Work out the finished part from the listing and answer in its coordinate system (mm). Coordinates: 2 decimals unless noted, no trailing zeros. Write each loop counter-clockwise with the first axis right and the second up, starting at its lowest first coordinate (ties: lowest second). Pieces come first, ordered by that corner, then holes. Notation, with made-up numbers: M 89,-22.5 L 104,-22.5 A20 cw 104,-3.5 Z; hole C 33,85 d10. An arc over 180 degrees is marked long. Answer as CSV lines item,"result". Start each with the question number.
(1) A cutting plane is placed at D-D on x = 0. Give the vertices of the cut face in (y, z), then the cut area to 3 significant figures.
(2) A cutting plane is placed at B-B on y = 22.5. Give the vertices of the cut face in (x, z).
(3) A cutting plane is placed at C-C on z = 1. Count the separate pieces of the cut face and the enclosed holes in it, then the cut area to 3 significant figures.
(4) A cutting plane is placed at A-A on x = 15.5. Give the vertices of the cut face in (y, z).
(5) Find the intervals of material crossed by L1, parallel to X at y = 25, z = 0.15; L2, parallel to Y at x = 15.5, z = 0.9; L3, parallel to Y at x = -25.5, z = 1.95, in increasing order. Write a range as [from, to].
(6) A flat-ended cylindrical pin translates along its axis: P1, Ø2, axis at x = 15.5, y = 15.5, coming from the +Z side. Find the tip coordinate at first contact, or state that the pin passes through.
from build123d import *

# Parameters (mm, degrees)
SKIZZE1_W                        = 70
SKIZZE1_H                        = 70
AUFSATZ_LINEAR_AUSTRAGEN1_DEPTH  = 2
VERRUNDUNG2_R                    = 2
F_23_0_23_DURCHMESSER_BOHRUNG1_D = 23
DURCHGANGSLOCH_F_R_M31_D         = 3.4
SCHNITT_LINEAR_AUSTRAGEN1_DEPTH  = 50.537864306


with BuildPart() as part:
    # Skizze1 → Aufsatz-Linear austragen1 (new body)
    with BuildSketch(Plane.XY):
        Rectangle(SKIZZE1_W, SKIZZE1_H)
    extrude(amount=AUFSATZ_LINEAR_AUSTRAGEN1_DEPTH)

    # Verrundung2
    verrundung2_edges = [part.edges().sort_by_distance(p)[0] for p in [
        (-35, 35, 1),
        (35, 35, 1),
        (35, -35, 1),
        (-35, -35, 1),
    ]]
    fillet(verrundung2_edges, radius=VERRUNDUNG2_R)

    # Ø23.0 (23) Durchmesser Bohrung1 (through all)
    with Locations(Plane.XY.offset(2)):
        with Locations((0, 0)):
            Hole(F_23_0_23_DURCHMESSER_BOHRUNG1_D / 2)

    # Durchgangsloch für M31 (through all)
    with Locations(Plane.XY.offset(2)):
        with Locations((-15.5, 15.5), (15.5, 15.5), (15.5, -15.5), (-15.5, -15.5)):
            Hole(DURCHGANGSLOCH_F_R_M31_D / 2)

    # Skizze8 → Schnitt-Linear austragen1 (cut, through all)
    with BuildSketch(Plane.XY.offset(2)):
        with BuildLine():
            Line((-26.5, 30), (-26.5, 10))
            ThreePointArc((-26.5, 10), (-25, 8.5), (-23.5, 10))
            Line((-23.5, 10), (-23.5, 30))
            ThreePointArc((-23.5, 30), (-25, 31.5), (-26.5, 30))
        make_face()
        with BuildLine():
            Line((-26.5, -10), (-26.5, -30))
            ThreePointArc((-26.5, -30), (-25, -31.5), (-23.5, -30))
            Line((-23.5, -30), (-23.5, -10))
            ThreePointArc((-23.5, -10), (-25, -8.5), (-26.5, -10))
        make_face()
        with BuildLine():
            Line((23.5, -10), (23.5, -30))
            ThreePointArc((23.5, -30), (25, -31.5), (26.5, -30))
            Line((26.5, -30), (26.5, -10))
            ThreePointArc((26.5, -10), (25, -8.5), (23.5, -10))
        make_face()
        with BuildLine():
            Line((23.5, 30), (23.5, 10))
            ThreePointArc((23.5, 10), (25, 8.5), (26.5, 10))
            Line((26.5, 10), (26.5, 30))
            ThreePointArc((26.5, 30), (25, 31.5), (23.5, 30))
        make_face()
    extrude(amount=-SCHNITT_LINEAR_AUSTRAGEN1_DEPTH, mode=Mode.SUBTRACT)


solid = part.part
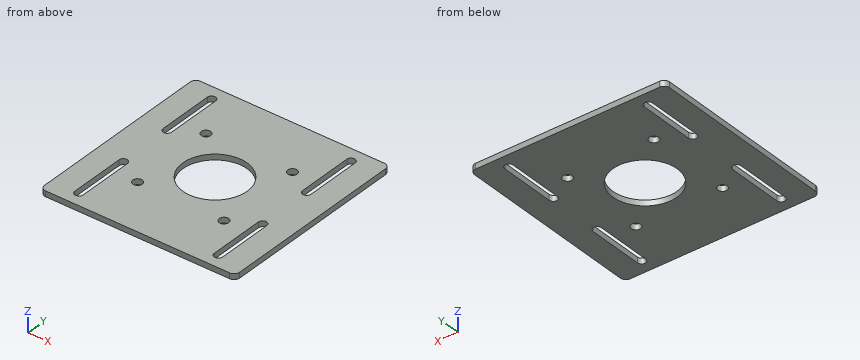
Here are the results:
1,outline,"M -35,0 L -11.5,0 L -11.5,2 L -35,2 Z; M 11.5,0 L 35,0 L 35,2 L 11.5,2 Z"
1,area,"94.0 mm^2"
2,outline,"M -35,0 L -26.5,0 L -26.5,2 L -35,2 Z; M -23.5,0 L 23.5,0 L 23.5,2 L -23.5,2 Z; M 26.5,0 L 35,0 L 35,2 L 26.5,2 Z"
3,separate pieces,"1"
3,enclosed holes,"9"
3,area,"4,180 mm^2"
4,outline,"M -35,0 L -17.2,0 L -17.2,2 L -35,2 Z; M -13.8,0 L 13.8,0 L 13.8,2 L -13.8,2 Z; M 17.2,0 L 35,0 L 35,2 L 17.2,2 Z"
5,L1,"x = [-35, -26.5], [-23.5, 23.5], [26.5, 35]"
5,L2,"y = [-35, -17.2], [-13.8, 13.8], [17.2, 35]"
5,L3,"y = [-35, -31.41], [-8.59, 8.59], [31.41, 35]"
6,P1,"passes through"
